```python
from build123d import *

# Parameters (mm, degrees)
EXTRUDE_1_DEPTH     = 50
SKETCH_2_R          = 2.6
CUT_EXTRUDE_1_DEPTH = 51
SKETCH_3_R          = 2.6
EXTRUDE_2_DEPTH     = 47


with BuildPart() as part:
    # 草图1 → 凸台-拉伸1 (new body)
    with BuildSketch(Plane(origin=(0, 0, 0), x_dir=(1, 0, 0), z_dir=(0, 1, 0))):
        Polygon((4.041451884, 0), (2.020725942, 3.5), (-2.020725942, 3.5), (-4.041451884, 0), (-2.020725942, -3.5), (2.020725942, -3.5), align=None)
    extrude(amount=EXTRUDE_1_DEPTH)

    # 草图2 → 切除-拉伸1 (cut, through all)
    with BuildSketch(Plane(origin=(0, 50, 0), x_dir=(1, 0, 0), z_dir=(0, 1, 0))):
        Circle(SKETCH_2_R)
    extrude(amount=-CUT_EXTRUDE_1_DEPTH, mode=Mode.SUBTRACT)

    # 草图3 → 凸台-拉伸2 (add)
    with BuildSketch(Plane(origin=(0, 10, 0), x_dir=(-1, 0, 0), z_dir=(0, -1, 0))):
        Circle(SKETCH_3_R)
    extrude(amount=-EXTRUDE_2_DEPTH)


solid = part.part
```
The listing builds one solid part. Answer for the finished solid, in the listing's coordinates (mm). A direction names the side the tool comes from. Round coordinates to 2 decimals unless told otherwise and drop trailing zeros. Loops run counter-clockwise (first coordinate to the right, second up) from the corner with the lowest first, then second, coordinate; pieces in that order, holes last.
Q1. Given pin 1 Ø4 at (x, z) = (0, 0.5) entering from -Y, flat-ended and moving along its own axis, determine where the tip first touches the part or whether it passes through.
Q2. Section A-A, the plane y = 9.5 is taken. Determine the outline of the cut face in (x, z).
Q3. Section B-B, the plane x = 0 is taken. Determine the outline of the cut face in (y, z).
Q4. Section C-C, the plane z = 1.25 is taken. Determine the outline of the cut face in (x, y).
Q5. Find the intervals of material crossed by line 1 (Z direction, x = 0, y = 8); line 2 (X direction, y = 3.25, z = 0); line 3 (Y direction, x = 0, z = -3), in increasing order.
Q6. Which of the six approach directions +Z, -Z, +X, -X, +Y, -Y give full straight-line access (tool end or side, diameter ignored) to faces 4 (the face through (3, 50, 0)), 5 (the face through (-3, 24.6, -1.8)), 6 (the face through (0, 10, 0))?
Q7. For a pull along X with two mould halves and no side action, classify faces 1 (the face through (3, 0, 0)), 2 (the face through (3, 24.6, 1.8)), 3 (the face through (-0.338, 5.07, -2.578)) as released by +X, released by -X, zero draft, split by the parting line, or undercut.
Q8. Section D-D, the plane y = 39 is taken. Determine the outline of the cut face in (x, z).
Completed:
1. pin 1: stops at y = 10
2. outline: (-4.04, 0) - (-2.02, -3.5) - (2.02, -3.5) - (4.04, 0) - (2.02, 3.5) - (-2.02, 3.5) - close; hole circle Ø5.2 at (0, 0)
3. outline: (0, -3.5) - (50, -3.5) - (50, -2.6) - (57, -2.6) - (57, 2.6) - (50, 2.6) - (50, 3.5) - (0, 3.5) - (0, 2.6) - (10, 2.6) - (10, -2.6) - (0, -2.6) - close
4. outline: (-3.32, 0) - (-2.28, 0) - (-2.28, 10) - (2.28, 10) - (2.28, 0) - (3.32, 0) - (3.32, 50) - (2.28, 50) - (2.28, 57) - (-2.28, 57) - (-2.28, 50) - (-3.32, 50) - close
5. line 1: z = -3.5 to -2.6, 2.6 to 3.5
5. line 2: x = -4.04 to -2.6, 2.6 to 4.04
5. line 3: y = 0 to 50
6. face 4: +Y
6. face 5: -Z, -X, +Y, -Y
6. face 6: -Y
7. face 1: zero draft
7. face 2: released by +X
7. face 3: undercut
8. outline: (-4.04, 0) - (-2.02, -3.5) - (2.02, -3.5) - (4.04, 0) - (2.02, 3.5) - (-2.02, 3.5) - close
